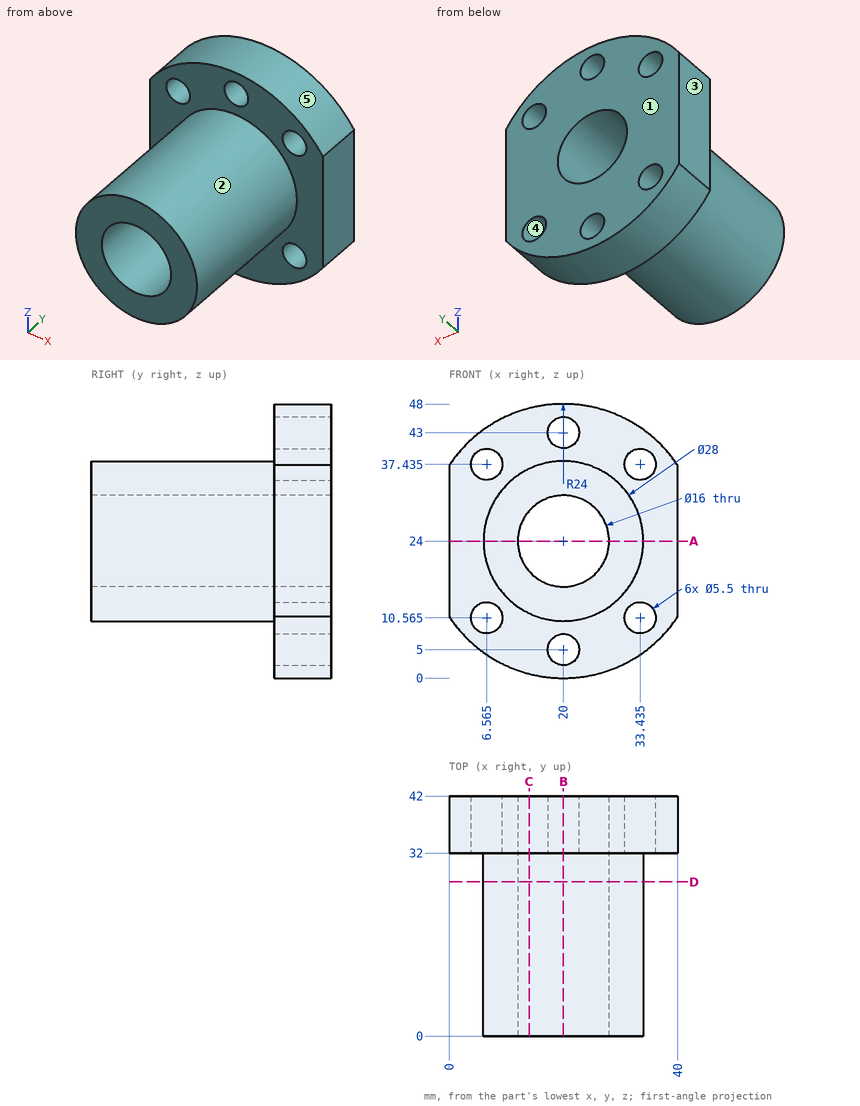
Print and shaded views of the part. All mm, measured from the part's lowest x, y and z. A direction names the side the tool comes from. Coordinates: 2 decimals unless noted, no trailing zeros. Write each loop counter-clockwise with the first axis right and the second up, starting at its lowest first coordinate (ties: lowest second). Pieces come first, ordered by that corner, then holes.
(1) Two-plate mould, pull along Z, no slides. Class the marked faces 3, 4 and 5: +Z half, -Z half, draft (parallel to the pull), parting line (faces both ways), or undercut.
(2) Cut at C-C, the plane x = 14. List the corners of the cut face in (y, z), and give its area (3 significant figures).
(3) Flat gauge pins, fed straight in: pin 1 (9.5 mm diameter, centred on x = 20, z = 24, fed in from +Y); pin 2 (10 mm diameter, centred on x = 28.5, y = 19.5, fed in from -Z); pin 3 (9 mm diameter, centred on x = 33.44, z = 37.44, fed in from -Y); pin 4 (5 mm diameter, centred on x = 10.5, y = 34, fed in from -Z). Where does each tip first touch, or does it go through?
(4) Cut at A-A, the plane z = 24. List the corners of the cut face in (x, y), and give its area (3 significant figures).
(5) Drill centre lines: probe 1 along Z at (x, y) = (19.5, 37); probe 2 along Y at (x, z) = (36.5, 16.5); probe 3 along X at (y, z) = (38, 8.5). Where is each one in solid material? Low to high.
(6) Cut at D-D, the plane y = 27. List the corners of the cut face in (x, z), and give its area (3 significant figures).
(7) Cut at B-B, the plane x = 20. List the corners of the cut face in (y, z).
(8) 3-axis set-ups, long thin cutter, end or side, ignore diameter. For the marked faces 1 and 2: which of +Z, -Z, +X, -X, +Y, -Y reach the whole face in a straight line?
Geometry says:
1. face 3: draft
1. face 4: undercut
1. face 5: +Z half
2. outline: (0, 11.35) - (32, 11.35) - (32, 0.76) - (42, 0.76) - (42, 18.71) - (0, 18.71) - close; (0, 29.29) - (42, 29.29) - (42, 47.24) - (32, 47.24) - (32, 36.65) - (0, 36.65) - close
2. area: 830 mm2
3. pin 1: passes through
3. pin 2: stops at z = 10.44
3. pin 3: stops at y = 32
3. pin 4: stops at z = 1.04
4. outline: (0, 32) - (6, 32) - (6, 0) - (12, 0) - (12, 42) - (0, 42) - close; (28, 0) - (34, 0) - (34, 32) - (40, 32) - (40, 42) - (28, 42) - close
4. area: 624 mm2
5. probe 1: z = 0.01 to 2.3, 7.7 to 16.02, 31.98 to 40.3, 45.7 to 47.99
5. probe 2: y = 32 to 42
5. probe 3: x = 1.68 to 4.75, 8.38 to 31.62, 35.25 to 38.32
6. outline: circle Ø28 at (20, 24); hole circle Ø16 at (20, 24)
6. area: 415 mm2
7. outline: (0, 10) - (32, 10) - (32, 7.75) - (42, 7.75) - (42, 16) - (0, 16) - close; (0, 32) - (42, 32) - (42, 40.25) - (32, 40.25) - (32, 38) - (0, 38) - close; (32, 0) - (42, 0) - (42, 2.25) - (32, 2.25) - close; (32, 45.75) - (42, 45.75) - (42, 48) - (32, 48) - close
8. face 1: +Z, -Z, +X, -X, +Y
8. face 2: -Y
